Work out the finished part from the listing and answer in its coordinate system (mm). Face numbers are marked on the shaded views. A direction names the side the tool comes from. Round coordinates to 2 decimals unless told otherwise and drop trailing zeros. Order: outer loops, then holes, each group sorted by start corner. A loop starts at its lowest first (then second) coordinate and runs counter-clockwise, first axis right, second up. Notation, with made-up numbers: (5, -21.75) -> (22, -21.75) arc R36 ccw to (22, 15.25) -> close; hole circle Ø11 at (89, 18). An arc over 180 degrees is marked (long way). Use one line per item in the form item = value.
```python
from build123d import *

# Parameters (mm, degrees)
SKETCH_315_R        = 3.237023897
SKETCH_315_R_2      = 1.631949552
SKETCH_315_R_3      = 1.631949719
EXTRUDE_1058_DEPTH  = 13.081
SKETCH_4_R          = 7.758938489
SKETCH_4_R_2        = 1.631949552
SKETCH_4_R_3        = 1.631949719
SKETCH_4_R_4        = 3.237023897
CUT_EXTRUDE_3_DEPTH = 5.588
SKETCH_4_2_R        = 7.758938489
SKETCH_5_R          = 3.237023897


with BuildPart() as part:
    # Sketch 315 → Extrude 1058 (new body)
    with BuildSketch(Plane(origin=(0, 0, 0), x_dir=(1, 0, 0), z_dir=(0, 1, 0))):
        with BuildLine():
            Line((0, -9.525000572), (0, -19.050001144))
            ThreePointArc((0, -19.050001144), (9.525002003, -28.575000286), (19.050001144, -19.049998283))
            Line((19.050001144, -19.049998283), (19.050001144, -9.525000572))
            ThreePointArc((19.050001144, -9.525000572), (9.525000572, 0), (0, -9.525000572))
        make_face()
        with Locations(Location((9.525000572, -9.525000572, 0), (0, 0, 270))):
            Circle(SKETCH_315_R, mode=Mode.SUBTRACT)
        with Locations(Location((3.175000612, -19.049999854, 0), (0, 0, 270))):
            Circle(SKETCH_315_R_2, mode=Mode.SUBTRACT)
        with Locations(Location((15.874999739, -19.050000406, 0), (0, 0, 270))):
            Circle(SKETCH_315_R_3, mode=Mode.SUBTRACT)
    extrude(amount=EXTRUDE_1058_DEPTH)

    # Sketch 4 → 拉伸3 (cut)
    # profile 1 of 2: a face of its own
    with BuildSketch(Plane(origin=(0, 0, 0), x_dir=(1, 0, 0), z_dir=(0, 1, 0))):
        with BuildLine():
            Line((0, -9.525000572), (0, -19.050001144))
            ThreePointArc((0, -19.050001144), (9.525002003, -28.575000286), (19.050001144, -19.049998283))
            Line((19.050001144, -19.049998283), (19.050001144, -9.525000572))
            ThreePointArc((19.050001144, -9.525000572), (9.525000572, 0), (0, -9.525000572))
        make_face()
        with Locations(Location((9.525000572, -9.525000572, 0), (0, 0, 270))):
            Circle(SKETCH_4_R, mode=Mode.SUBTRACT)
        with Locations(Location((3.175000612, -19.049999854, 0), (0, 0, 270))):
            Circle(SKETCH_4_R_2, mode=Mode.SUBTRACT)
        with Locations(Location((15.874999739, -19.050000406, 0), (0, 0, 270))):
            Circle(SKETCH_4_R_3, mode=Mode.SUBTRACT)
    # profile 2 of 2: a face of its own
    with BuildSketch(Plane(origin=(0, 0, 0), x_dir=(1, 0, 0), z_dir=(0, 1, 0))):
        with Locations(Location((9.525000572, -9.525000572, 0), (0, 0, 270))):
            Circle(SKETCH_4_R_4)
    extrude(amount=CUT_EXTRUDE_3_DEPTH, mode=Mode.SUBTRACT)

    # Sketch 4 2 → 切除-放样1 section 0
    with BuildSketch(Plane(origin=(0, 13.081000328, 0), x_dir=(1, 0, 0), z_dir=(0, 1, 0))):
        with Locations((9.525000572, -9.525000572)):
            Circle(SKETCH_4_2_R)
    # 草图5 → 切除-放样1 section 1
    with BuildSketch(Plane.XZ.offset(-5.588000298)):
        with Locations((9.525000572, 9.525000572)):
            Circle(SKETCH_5_R)
    loft(mode=Mode.SUBTRACT)


solid = part.part
```
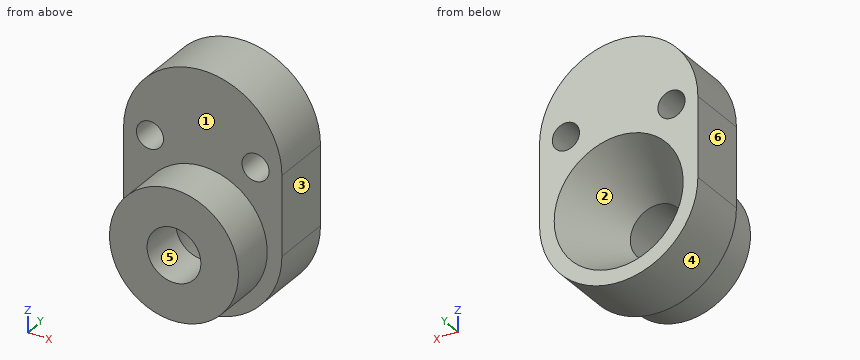
Item 1: Consider line 1 along Z through (x, y) = (3.25, 12.75); line 2 along X through (y, z) = (12.5, 20); line 3 along X through (y, z) = (9.5, 17.75). Determine where each line is inside the solid, lowest interval first.
Findings:
line_1 = 2.36 to 5.31, 13.74 to 17.42, 20.68 to 26.22
line_2 = 0.05 to 1.85, 4.5 to 14.55, 17.2 to 19
line_3 = 0 to 2.19, 4.16 to 14.89, 16.86 to 19.05
Item 2: Determine the mould class of the marked faces 3, 4, 5 and 6 for opening direction X: released by +X, released by -X, zero draft, split by the parting line, or undercut.
Findings:
face_3 = released by +X
face_4 = split by the parting line
face_5 = undercut
face_6 = released by -X
Item 3: The part is cut by section C-C, the plane z = 26.25. Give the vertices of the cut face in (x, y), and give its area (4 significant figures).
Findings:
outline = (3.29, 5.59) -> (15.76, 5.59) -> (15.76, 13.08) -> (3.29, 13.08) -> close
area = 93.45 mm^2
Item 4: For the marked faces 1 and 2, determine the directions among +Z, -Z, +X, -X, +Y, -Y from which every point of the face is accessible in a straight line to the end or side of a thin tool.
Findings:
face_1 = -Y
face_2 = +Y
Item 5: The part is cut by section A-A, the plane y = 9.75. Give the vertices of the cut face in (x, z) (3 decimals).
Findings:
outline = (0, 9.525) arc R9.525 ccw to (19.05, 9.525) -> (19.05, 19.05) arc R9.525 ccw to (0, 19.05) -> close; hole circle Ø3.264 at (3.175, 19.05); hole circle Ø11.497 at (9.525, 9.525); hole circle Ø3.264 at (15.875, 19.05)
Item 6: Flat-ended cylindrical pins translate along their axes: P1, Ø1.5, axis at x = 13, y = 4, coming from the +Z side; P2, Ø4, axis at x = 2.5, y = 9.5, coming from the -Z side; P3, Ø6, axis at x = 9, z = 7, coming from the +Y side; P4, Ø2.5, axis at x = 3.175, z = 19.05, coming from the +Y side. Find the tip coordinate at first contact, or state that the pin passes through.
Findings:
P1 = 16.79
P2 = 1.43
P3 = 9.47
P4 = through
Item 7: The part is cut by section B-B, the plane z = 18. Give the vertices of the cut face in (x, y).
Findings:
outline = (0, 5.59) -> (1.93, 5.59) -> (1.93, 13.08) -> (0, 13.08) -> close; (4.42, 5.59) -> (14.63, 5.59) -> (14.63, 13.08) -> (4.42, 13.08) -> close; (17.12, 5.59) -> (19.05, 5.59) -> (19.05, 13.08) -> (17.12, 13.08) -> close
